Here's how the part is built. I have some questions about the finished solid (model axes, mm). Coordinates: 2 decimals unless noted, no trailing zeros. Write each loop counter-clockwise with the first axis right and the second up, starting at its lowest first coordinate (ties: lowest second). Pieces come first, ordered by that corner, then holes. Notation, with made-up numbers: (88, 56.5) -> (145, 56.5) arc R20 ccw to (145, 90.5) -> close; hole circle Ø8 at (-1, 38.25). An arc over 180 degrees is marked (long way). Put each result on its own line as item: value. Start each with the question number.
Item 1: I need wall thicknesses on line 1 (Y direction, x = 1.3, z = -8); line 2 (Y direction, x = 0.65, z = -39); line 3 (Y direction, x = 2.15, z = -23). Which ranges of each line are inside material? Lowest first, please. Write a range as [from, to].
Item 2: I want a section at B-B, the plane y = 20. List the corners of the cut face in (x, z) for me.
Item 3: If we mould it in two halves opening along Y, with no side actions, what happens to faces 1 (the face through (1, 25, -22)), 2 (the face through (1.48, 22.11, -9.34)), 3 (the face through (1, 18, -39)), 4 (the face through (3, 0, -17))? For each: released by +Y, released by -Y, zero draft, split by the parting line, or undercut.
Item 4: I want a section at A-A, the plane z = -8. List the corners of the cut face in (x, y) for me, then the cut area to 3 significant figures.
Item 5: I want a section at D-D, the plane z = -27. List the corners of the cut face in (x, y) for me.
Item 6: I want a section at C-C, the plane z = -39. List the corners of the cut face in (x, y) for me, then the cut area to 3 significant figures.
from build123d import *

# Parameters (mm, degrees)
ESQUISSE1_R        = 2
ESQUISSE1_R_2      = 2.5
BOSS_EXTRU_1_DEPTH = 3
CONG_1_R           = 4


with BuildPart() as part:
    # Esquisse1 → Boss.-Extru.1 (new body)
    with BuildSketch(Plane(origin=(0, 0, 0), x_dir=(0, 0, -1), z_dir=(1, 0, 0))):
        with BuildLine():
            Line((0, 25), (44, 25))
            Line((44, 25), (44, 11.728704106))
            ThreePointArc((44, 11.728704106), (26.25, 0), (44, -11.728704106))
            Line((44, -11.728704106), (44, -25))
            Line((44, -25), (0, -25))
            Line((0, -25), (0, 25))
        make_face()
        with Locations((39, 16)):
            Circle(ESQUISSE1_R, mode=Mode.SUBTRACT)
        with Locations((23, 0)):
            Circle(ESQUISSE1_R, mode=Mode.SUBTRACT)
        with Locations(Location((39, -16, 0), (0, 0, 180))):
            Circle(ESQUISSE1_R, mode=Mode.SUBTRACT)
        with Locations((8, 20)):
            Circle(ESQUISSE1_R_2, mode=Mode.SUBTRACT)
        with Locations(Location((8, -20, 0), (0, 0, 180))):
            Circle(ESQUISSE1_R_2, mode=Mode.SUBTRACT)
    extrude(amount=BOSS_EXTRU_1_DEPTH)

    # Congé1
    cong_1_edges = [part.edges().sort_by_distance(p)[0] for p in [
        (1.5, 25, 0),
        (1.5, 25, -44),
        (1.5, 11.728704106, -44),
        (1.5, -11.728704106, -44),
        (1.5, -25, -44),
        (1.5, -25, 0),
    ]]
    fillet(cong_1_edges, radius=CONG_1_R)


solid = part.part
Calculated:
1. line 1: y = [-25, -22.5], [-17.5, 17.5], [22.5, 25]
1. line 2: y = [-25, -18], [-14, -12.75], [12.75, 14], [18, 25]
1. line 3: y = [-25, -2], [2, 25]
2. outline: (0, -44) -> (3, -44) -> (3, -10.5) -> (0, -10.5) -> close; (0, -5.5) -> (3, -5.5) -> (3, 0) -> (0, 0) -> close
3. face 1: released by +Y
3. face 2: undercut
3. face 3: undercut
3. face 4: zero draft
4. outline: (0, -25) -> (3, -25) -> (3, -22.5) -> (0, -22.5) -> close; (0, -17.5) -> (3, -17.5) -> (3, 17.5) -> (0, 17.5) -> close; (0, 22.5) -> (3, 22.5) -> (3, 25) -> (0, 25) -> close
4. area: 120 mm2
5. outline: (0, -25) -> (3, -25) -> (3, -4.31) -> (0, -4.31) -> close; (0, 4.31) -> (3, 4.31) -> (3, 25) -> (0, 25) -> close
6. outline: (0, -25) -> (3, -25) -> (3, -18) -> (0, -18) -> close; (0, -14) -> (3, -14) -> (3, -12.75) -> (0, -12.75) -> close; (0, 12.75) -> (3, 12.75) -> (3, 14) -> (0, 14) -> close; (0, 18) -> (3, 18) -> (3, 25) -> (0, 25) -> close
6. area: 49.5 mm2
